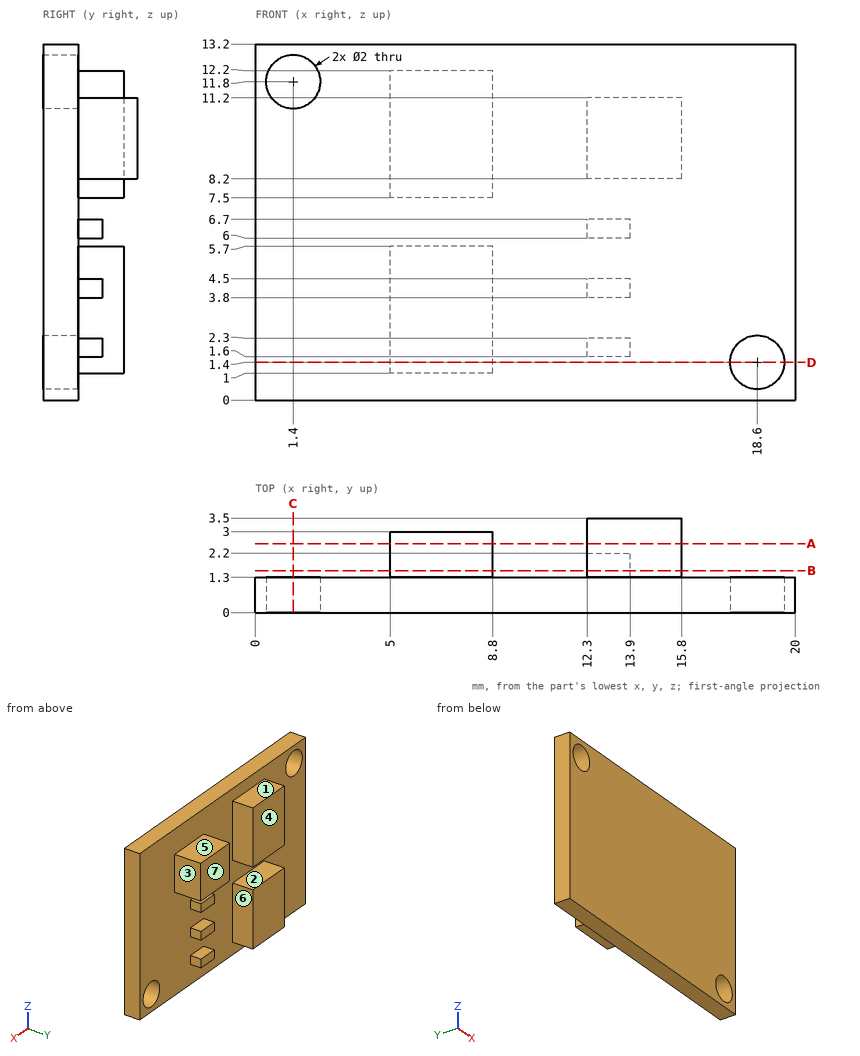
Here's the drawing with two shaded views (mm, measured from the low corner). I have some questions. A direction names the side the tool comes from. Give positions to 0.01 mm unless a question says otherwise; leave off trailing zeros. Loops run counter-clockwise (first coordinate to the right, second up) from the corner with the lowest first, then second, coordinate; pieces in that order, holes last. Notation, with made-up numbers: (15.25, -29) -> (24.25, -29) arc R19 cw to (24.25, -7) -> close; hole circle Ø4 at (82, 58). An arc over 180 degrees is marked (long way). Answer as a JSON object with one key per item and string values. Group by question number.
Item 1: Will these pins go through, and if not, where does the flat tip stop? pin 1 (0.7 mm diameter, centred on x = 13.5, y = 2, fed in from +Z); pin 2 (1 mm diameter, centred on x = 12.5, y = 2, fed in from -Z); pin 3 (6 mm diameter, centred on x = 11.5, z = 2.5, fed in from -Y); pin 4 (4 mm diameter, centred on x = 13.5, z = 5, fed in from +Y).
Item 2: On a 3-axis mill with a long thin cutter (end or side, diameter ignored), from which of +Z, -Z, +X, -X, +Y, -Y can I reach the whole of each face in a straight line? I mean the marked faces 4, 5, 6 and 7. Say none if no direction works.
Item 3: Imagine slicing it at C-C on x = 1.4. Write out the boundary of the cut face in (y, z), then the cut area to 3 significant figures.
Item 4: Imagine slicing it at B-B on y = 1.55. Write out the boundary of the cut face in (x, z).
Item 5: Imagine slicing it at A-A on y = 2.55. Write out the boundary of the cut face in (x, z), then the cut area to 3 significant figures.
Item 6: Imagine slicing it at D-D on z = 1.4. Write out the boundary of the cut face in (x, y).
Item 7: I need wall thicknesses on L1, parallel to Z at x = 18.6, y = 1; L2, parallel to Z at x = 6.75, y = 2.55; L3, parallel to X at y = 1.05, z = 1.4. Which ranges of each line are inside material? Lowest first, please.
Item 8: Thinking about a two-plate mould opening in Z: for the marked faces 1, 2 and 3, which applies, pulls with the +Z half, pulls with the -Z half, needs draft (parallel to the pull), parting line crosses it, or undercut?
Answer list:
{
 "1": {"pin 1": "stops at z = 11.2", "pin 2": "stops at z = 1.6", "pin 3": "stops at y = 0", "pin 4": "stops at y = 2.2"},
 "2": {"face 4": "+Z, -Z, -X, +Y", "face 5": "+Z, +X, +Y", "face 6": "+Z, -Z, +Y", "face 7": "+Z, -Z, +X, -X, +Y"},
 "3": {"outline": "(0, 0) -> (1.3, 0) -> (1.3, 10.8) -> (0, 10.8) -> close; (0, 12.8) -> (1.3, 12.8) -> (1.3, 13.2) -> (0, 13.2) -> close", "area": "14.6 mm2"},
 "4": {"outline": "(5, 1) -> (8.8, 1) -> (8.8, 5.7) -> (5, 5.7) -> close; (5, 7.5) -> (8.8, 7.5) -> (8.8, 12.2) -> (5, 12.2) -> close; (12.3, 1.6) -> (13.9, 1.6) -> (13.9, 2.3) -> (12.3, 2.3) -> close; (12.3, 3.8) -> (13.9, 3.8) -> (13.9, 4.5) -> (12.3, 4.5) -> close; (12.3, 6) -> (13.9, 6) -> (13.9, 6.7) -> (12.3, 6.7) -> close; (12.3, 8.2) -> (15.8, 8.2) -> (15.8, 11.2) -> (12.3, 11.2) -> close"},
 "5": {"outline": "(5, 1) -> (8.8, 1) -> (8.8, 5.7) -> (5, 5.7) -> close; (5, 7.5) -> (8.8, 7.5) -> (8.8, 12.2) -> (5, 12.2) -> close; (12.3, 8.2) -> (15.8, 8.2) -> (15.8, 11.2) -> (12.3, 11.2) -> close", "area": "46.2 mm2"},
 "6": {"outline": "(0, 0) -> (17.6, 0) -> (17.6, 1.3) -> (8.8, 1.3) -> (8.8, 3) -> (5, 3) -> (5, 1.3) -> (0, 1.3) -> close; (19.6, 0) -> (20, 0) -> (20, 1.3) -> (19.6, 1.3) -> close"},
 "7": {"L1": "z = 0 to 0.4, 2.4 to 13.2", "L2": "z = 1 to 5.7, 7.5 to 12.2", "L3": "x = 0 to 17.6, 19.6 to 20"},
 "8": {"face 1": "pulls with the +Z half", "face 2": "undercut", "face 3": "needs draft"}
}
